```python
from build123d import *

# Parameters (mm, degrees)
SKETCH1_W           = 40
SKETCH1_H           = 240
BOSS_EXTRUDE2_DEPTH = 4
SKETCH2_W           = 40
SKETCH2_H           = 240
SKETCH2_W_2         = 36
SKETCH2_H_2         = 236
BOSS_EXTRUDE4_DEPTH = 45
SKETCH3_W           = 14
SKETCH3_H           = 14
BOSS_EXTRUDE5_DEPTH = 45
SKETCH4_R           = 1.75
CUT_EXTRUDE1_DEPTH  = 90
FILLET1_R           = 10
FILLET2_R           = 10
SKETCH5_R           = 3.5
CUT_EXTRUDE2_DEPTH  = 45
SKETCH6_W           = 20
SKETCH6_H           = 10
CUT_EXTRUDE3_DEPTH  = 10
SKETCH7_W           = 75
SKETCH7_H           = 49
BOSS_EXTRUDE6_DEPTH = 45
SKETCH8_W           = 45
SKETCH8_H           = 71
CUT_EXTRUDE4_DEPTH  = 45
SKETCH9_W           = 36
SKETCH9_H           = 4
CUT_EXTRUDE5_DEPTH  = 50


with BuildPart() as part:
    # Sketch1 → Boss-Extrude2 (new body)
    with BuildSketch(Plane(origin=(0, 0, 0), x_dir=(1, 0, 0), z_dir=(0, 1, 0))):
        Rectangle(SKETCH1_W, SKETCH1_H)
    extrude(amount=BOSS_EXTRUDE2_DEPTH)

    # Sketch2 → Boss-Extrude4 (add)
    with BuildSketch(Plane(origin=(0, 4, 0), x_dir=(1, 0, 0), z_dir=(0, 1, 0))):
        Rectangle(SKETCH2_W, SKETCH2_H)
        Rectangle(SKETCH2_W_2, SKETCH2_H_2, mode=Mode.SUBTRACT)
    extrude(amount=BOSS_EXTRUDE4_DEPTH)

    # Sketch3 → Boss-Extrude5 (add)
    with BuildSketch(Plane(origin=(0, 4, 0), x_dir=(1, 0, 0), z_dir=(0, 1, 0))):
        with Locations((-11, 111)):
            Rectangle(SKETCH3_W, SKETCH3_H)
        with Locations((11, 111)):
            Rectangle(SKETCH3_W, SKETCH3_H)
        with Locations((-11, -111)):
            Rectangle(SKETCH3_W, SKETCH3_H)
        with Locations((11, -111)):
            Rectangle(SKETCH3_W, SKETCH3_H)
    extrude(amount=BOSS_EXTRUDE5_DEPTH)

    # Sketch4 → Cut-Extrude1 (cut)
    with BuildSketch(Plane(origin=(0, 0, 0), x_dir=(-1, 0, 0), z_dir=(0, -1, 0))):
        with Locations(Location((12, -112, 0), (0, 0, 90))):
            Circle(SKETCH4_R)
        with Locations(Location((-13, -112, 0), (0, 0, 90))):
            Circle(SKETCH4_R)
        with Locations(Location((12, 112, 0), (0, 0, 90))):
            Circle(SKETCH4_R)
        with Locations(Location((-13, 112, 0), (0, 0, 90))):
            Circle(SKETCH4_R)
    extrude(amount=-CUT_EXTRUDE1_DEPTH, mode=Mode.SUBTRACT)

    # Fillet1
    fillet1_edges = [part.edges().sort_by_distance(p)[0] for p in [
        (-20, 24.5, -120),
    ]]
    fillet(fillet1_edges, radius=FILLET1_R)

    # Fillet2
    fillet2_edges = [part.edges().sort_by_distance(p)[0] for p in [
        (-20, 24.5, 120),
    ]]
    fillet(fillet2_edges, radius=FILLET2_R)

    # Sketch5 → Cut-Extrude2 (cut)
    with BuildSketch(Plane(origin=(0, 0, 0), x_dir=(-1, 0, 0), z_dir=(0, -1, 0))):
        with Locations(Location((12, -112, 0), (0, 0, 90))):
            Circle(SKETCH5_R)
        with Locations(Location((-13, -112, 0), (0, 0, 90))):
            Circle(SKETCH5_R)
        with Locations(Location((12, 112, 0), (0, 0, 90))):
            Circle(SKETCH5_R)
        with Locations(Location((-13, 112, 0), (0, 0, 90))):
            Circle(SKETCH5_R)
    extrude(amount=-CUT_EXTRUDE2_DEPTH, mode=Mode.SUBTRACT)

    # Sketch6 → Cut-Extrude3 (cut)
    with BuildSketch(Plane(origin=(20, 0, 0), x_dir=(0, 0, -1), z_dir=(1, 0, 0))):
        with Locations((0, 44)):
            Rectangle(SKETCH6_W, SKETCH6_H)
    extrude(amount=-CUT_EXTRUDE3_DEPTH, mode=Mode.SUBTRACT)

    # Sketch7 → Boss-Extrude6 (add)
    with BuildSketch(Plane(origin=(20, 0, 0), x_dir=(0, 0, -1), z_dir=(1, 0, 0))):
        with Locations((-82.5, 24.5)):
            Rectangle(SKETCH7_W, SKETCH7_H)
    extrude(amount=BOSS_EXTRUDE6_DEPTH)

    # Sketch8 → Cut-Extrude4 (cut)
    with BuildSketch(Plane(origin=(0, 49, 0), x_dir=(1, 0, 0), z_dir=(0, 1, 0))):
        with Locations((40.5, -82.5)):
            Rectangle(SKETCH8_W, SKETCH8_H)
    extrude(amount=-CUT_EXTRUDE4_DEPTH, mode=Mode.SUBTRACT)

    # Sketch9 → Cut-Extrude5 (cut)
    with BuildSketch(Plane(origin=(0, 49, 0), x_dir=(1, 0, 0), z_dir=(0, 1, 0))):
        with Locations((0, -106)):
            Rectangle(SKETCH9_W, SKETCH9_H)
    extrude(amount=-CUT_EXTRUDE5_DEPTH, mode=Mode.SUBTRACT)


solid = part.part
```
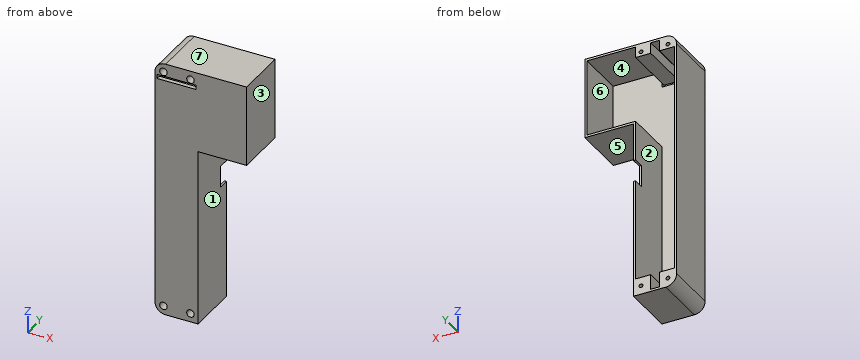
Source: CAD feature listing. Evaluate the final solid. Frame: model axes, mm. Face numbers are marked on the shaded views. A direction names the side the tool comes from. Give positions to 0.01 mm unless a question says otherwise; leave off trailing zeros. Write each loop counter-clockwise with the first axis right and the second up, starting at its lowest first coordinate (ties: lowest second). Pieces come first, ordered by that corner, then holes. Notation, with made-up numbers: (79.5, -6) - (136.5, -6) arc R31 cw to (136.5, 23) - close; hole circle Ø7 at (-25, 52.25). An arc over 180 degrees is marked (long way). One line per item, written item: value. Start each with the question number.
Q1. Material intervals for probe 1 along Z at (x, y) = (32, 41.5); probe 2 along X at (y, z) = (33, 74); probe 3 along X at (y, z) = (27, -53), sorted ascending. Write a range as from..to.
Q2. Draft query along Z for the marked faces 4, 5, 6 and 7. Return one class per face: +Z half, -Z half, draft (parallel to the pull), parting line (faces both ways), or undercut.
Q3. Section query B-B, the plane z = 3. Return the cut outline in (x, y), then the cut area to 3 significant figures.
Q4. Set-up query: the marked faces 1, 2 and 3. Return all of +Z, -Z, +X, -X, +Y, -Y with unobstructed straight access to the full face (end or side cutting, diameter ignored); none if empty.
Q5. Section query A-A, the plane y = 29.5. Return the cut outline in (x, z), then the cut area to 3 significant figures.
Q6. Section query C-C, the plane x = 53. Return the cut outline in (y, z).
Q7. First-contact query: pin 1 Ø7 at (y, z) = (36.5, -114.5) entering from -X; pin 2 Ø22.5 at (x, y) = (38, 22.5) entering from -Z; pin 3 Ø1.5 at (x, z) = (-0.5, 95.5) entering from +Y. Flat tips, straight axial feed; report the tip coordinate or a pass-through.
Answer:
1. probe 1: z = 45..47, 118..120
1. probe 2: x = -20..-18, 63..65
1. probe 3: x = -20..-18, 18..20
2. face 4: undercut
2. face 5: -Z half
2. face 6: undercut
2. face 7: +Z half
3. outline: (-20, 0) - (20, 0) - (20, 39) - (18, 39) - (18, 4) - (-18, 4) - (-18, 49) - (-20, 49) - close
3. area: 320 mm2
4. face 1: -Z, +X, +Y, -Y
4. face 2: +Y
4. face 3: +Z, -Z, +X, +Y, -Y
5. outline: (-20, -110) arc R10 ccw to (-10, -120) - (20, -120) - (20, 45) - (65, 45) - (65, 120) - (-10, 120) arc R10 ccw to (-20, 110) - close; hole (-18, -104) - (-4, -104) - (-4, -118) - (4, -118) - (4, -104) - (18, -104) - (18, 47) - (63, 47) - (63, 118) - (18, 118) - (18, 108) - (4, 108) - (4, 118) - (-4, 118) - (-4, 108) - (-18, 108) - close; hole circle Ø7 at (-12, -112); hole circle Ø7 at (-12, 112); hole circle Ø7 at (13, -112); hole circle Ø7 at (13, 112)
5. area: 1,760 mm2
6. outline: (0, 45) - (49, 45) - (49, 47) - (4, 47) - (4, 118) - (49, 118) - (49, 120) - (0, 120) - close
7. pin 1: stops at x = -19.95
7. pin 2: stops at z = 45
7. pin 3: stops at y = 4
